Here's how the part is built. I have some questions about the finished solid (model axes, mm). Face numbers are marked on the shaded views. A direction names the side the tool comes from. Round coordinates to 2 decimals unless told otherwise and drop trailing zeros. Loops run counter-clockwise (first coordinate to the right, second up) from the corner with the lowest first, then second, coordinate; pieces in that order, holes last. Notation, with made-up numbers: M 26.25,-7 L 77.25,-7 A23 cw 77.25,11 Z; hole C -8.5,70 d4. An arc over 180 degrees is marked long. Write item = value, one per line. Start each with the question number.
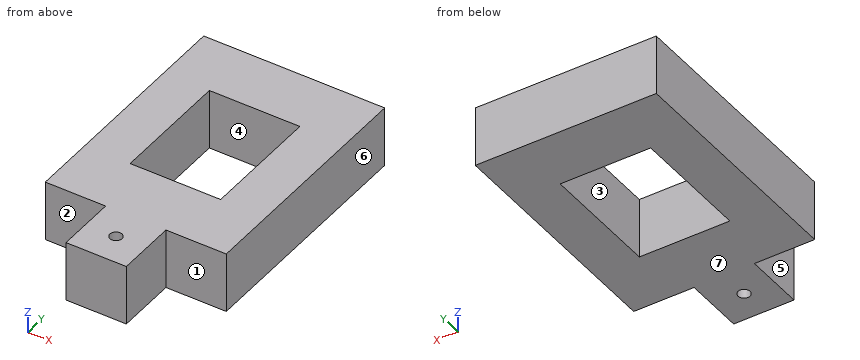
from build123d import *

# Parameters (mm, degrees)
SKETCH1_W           = 19.05
SKETCH1_H           = 31.75
BOSS_EXTRUDE1_DEPTH = 6.35
SKETCH2_W           = 9.525
SKETCH2_H           = 12.7
CUT_EXTRUDE1_DEPTH  = 6.35
SKETCH3_W           = 6.35
SKETCH3_H           = 6.35
CUT_EXTRUDE2_DEPTH  = 7.35
SKETCH4_R           = 0.635
CUT_EXTRUDE3_DEPTH  = 7.35


with BuildPart() as part:
    # Sketch1 → Boss-Extrude1 (new body)
    with BuildSketch(Plane.XY):
        with Locations((9.525, 15.875)):
            Rectangle(SKETCH1_W, SKETCH1_H)
    extrude(amount=BOSS_EXTRUDE1_DEPTH)

    # Sketch2 → Cut-Extrude1 (cut)
    with BuildSketch(Plane.XY.offset(6.35)):
        with Locations((9.525, 19.05)):
            Rectangle(SKETCH2_W, SKETCH2_H)
    extrude(amount=-CUT_EXTRUDE1_DEPTH, mode=Mode.SUBTRACT)

    # Sketch3 → Cut-Extrude2 (cut, through all)
    with BuildSketch(Plane(origin=(0, 0, 0), x_dir=(-1, 0, 0), z_dir=(0, 0, -1))):
        with Locations((-15.875, 3.175)):
            Rectangle(SKETCH3_W, SKETCH3_H)
        with Locations((-3.175, 3.175)):
            Rectangle(SKETCH3_W, SKETCH3_H)
    extrude(amount=-CUT_EXTRUDE2_DEPTH, mode=Mode.SUBTRACT)

    # Sketch4 → Cut-Extrude3 (cut, through all)
    with BuildSketch(Plane.XY.offset(6.35)):
        with Locations((9.525, 3.175)):
            Circle(SKETCH4_R)
    extrude(amount=-CUT_EXTRUDE3_DEPTH, mode=Mode.SUBTRACT)


solid = part.part
Item 1: I want a section at A-A, the plane x = 12. List the corners of the cut face in (y, z) for me.
Item 2: We'd pull the mould along X, two halves only. Please class the marked faces 4, 5, 6 and 7: released by +X, released by -X, zero draft, split by the parting line, or undercut.
Item 3: I want a section at C-C, the plane z = 1.25. State how many separate pieces and enclosed holes the cut face has, then the cut area to 3 significant figures.
Item 4: For the marked faces 1, 2 and 3, which set-ups out of +Z, -Z, +X, -X, +Y, -Y let a thin tool reach every point of the face, with its end or its side?
Item 5: Please list where these lines run through material, in increasing order: line 1 (X direction, y = 23.5, z = 4.5); line 2 (Y direction, x = 13.25, z = 5.25); line 3 (Y direction, x = 10, z = 5.5). Write a range as [from, to].
Item 6: I want a section at D-D, the plane x = 9.25. List the corners of the cut face in (y, z) for me.
Item 7: I want a section at B-B, the plane y = 24. List the corners of the cut face in (x, z) for me.
Item 8: Will these pins go through, and if not, where does the flat tip stop? pin 1 Ø0.8 at (x, y) = (9.525, 3.175) entering from -Z (3 decimals); pin 2 Ø3 at (x, z) = (17, 2) entering from -Y; pin 3 Ø3 at (y, z) = (4.5, 2) entering from -X.
Worked out:
q1.outline = M 0,0 L 12.7,0 L 12.7,6.35 L 0,6.35 Z; M 25.4,0 L 31.75,0 L 31.75,6.35 L 25.4,6.35 Z
q2.face_4 = undercut
q2.face_5 = released by -X
q2.face_6 = released by +X
q2.face_7 = zero draft
q3.separate_pieces = 1
q3.enclosed_holes = 2
q3.area = 402 mm2
q4.face_1 = +Z, -Z, +X, -Y
q4.face_2 = +Z, -Z, -X, -Y
q4.face_3 = +Z, -Z
q5.line_1 = [0, 4.76], [14.29, 19.05]
q5.line_2 = [6.35, 12.7], [25.4, 31.75]
q5.line_3 = [0, 2.75], [3.6, 12.7], [25.4, 31.75]
q6.outline = M 0,0 L 2.6,0 L 2.6,6.35 L 0,6.35 Z; M 3.75,0 L 12.7,0 L 12.7,6.35 L 3.75,6.35 Z; M 25.4,0 L 31.75,0 L 31.75,6.35 L 25.4,6.35 Z
q7.outline = M 0,0 L 4.76,0 L 4.76,6.35 L 0,6.35 Z; M 14.29,0 L 19.05,0 L 19.05,6.35 L 14.29,6.35 Z
q8.pin_1 = through
q8.pin_2 = 6.35
q8.pin_3 = 6.35
